```python
from build123d import *

# Parameters (mm, degrees)
F0_W     = 60
F0_H     = 9
F0_R     = 2
F1_DEPTH = 3
F3_DEPTH = 9
F5_DEPTH = 9


with BuildPart() as f1:
    # F0 (on Top) → F1 (new body)
    with BuildSketch(Plane.XY):
        Rectangle(F0_W, F0_H)
        with Locations((-14, 0)):
            Circle(F0_R, mode=Mode.SUBTRACT)
        with Locations((-7, 0)):
            Circle(F0_R, mode=Mode.SUBTRACT)
        Circle(F0_R, mode=Mode.SUBTRACT)
        with Locations((7, 0)):
            Circle(F0_R, mode=Mode.SUBTRACT)
        with Locations((14, 0)):
            Circle(F0_R, mode=Mode.SUBTRACT)
    extrude(amount=F1_DEPTH)

    # F2 (on face) → F3 (join)
    with BuildSketch(Plane(origin=(-30, 0, 0), x_dir=(0, -1, 0), z_dir=(-1, 0, 0))):
        with BuildLine():
            ThreePointArc((0, 0), (1.06066, 0.43934), (1.5, 1.5))
            ThreePointArc((1.5, 1.5), (1.06066, 2.56066), (0, 3))
            ThreePointArc((0, 3), (-1.5, 1.5), (0, 0))
        make_face()
    extrude(amount=F3_DEPTH)

    # F4 (on face) → F5 (join)
    with BuildSketch(Plane.YZ.offset(30)):
        with BuildLine():
            ThreePointArc((0, 0), (1.06066, 0.43934), (1.5, 1.5))
            ThreePointArc((1.5, 1.5), (1.06066, 2.56066), (0, 3))
            ThreePointArc((0, 3), (-1.5, 1.5), (0, 0))
        make_face()
    extrude(amount=F5_DEPTH)


solid = f1.part
```
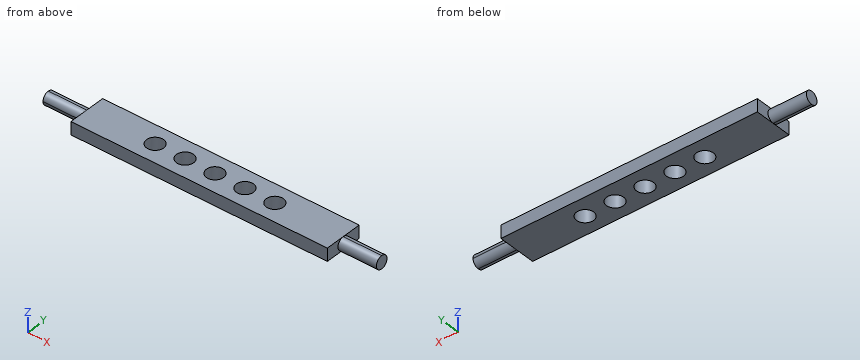
Part model, mm, in its own coordinate system. Round coordinates to 2 decimals unless told otherwise and drop trailing zeros. Loops run counter-clockwise (first coordinate to the right, second up) from the corner with the lowest first, then second, coordinate; pieces in that order, holes last.
1. Slice it at D-D (x = -33). Give the cut face in (y, z).
Solutions:
outline: circle Ø3 at (0, 1.5)
2. Flat gauge pin, fed straight in: pin 1 (5 mm diameter, centred on x = 14, y = 0, fed in from -Z). Where does the tip first touch, or does it go through?
Solutions:
pin 1: stops at z = 0
3. Slice it at A-A (x = -7). Give the cut face in (y, z).
Solutions:
outline: (-4.5, 0) - (-2, 0) - (-2, 3) - (-4.5, 3) - close; (2, 0) - (4.5, 0) - (4.5, 3) - (2, 3) - close
4. Slice it at C-C (y = -3.5). Give the cut face in (x, z).
Solutions:
outline: (-30, 0) - (30, 0) - (30, 3) - (-30, 3) - close
5. Drill centre lines: line 1 along X through (y, z) = (-0.25, 2.05); line 2 along Y through (x, z) = (14, 2.3); line 3 along X through (y, z) = (0.75, 2.5). Where is each one in solid material? Low to high.
Solutions:
line 1: x = -39 to -15.98, -12.02 to -8.98, -5.02 to -1.98, 1.98 to 5.02, 8.98 to 12.02, 15.98 to 39
line 2: y = -4.5 to -2, 2 to 4.5
line 3: x = -39 to -15.85, -12.15 to -8.85, -5.15 to -1.85, 1.85 to 5.15, 8.85 to 12.15, 15.85 to 39
6. Slice it at B-B (z = 0.6). Give the cut face in (x, y), and give its area (3 significant figures).
Solutions:
outline: (-39, -1.2) - (-30, -1.2) - (-30, -4.5) - (30, -4.5) - (30, -1.2) - (39, -1.2) - (39, 1.2) - (30, 1.2) - (30, 4.5) - (-30, 4.5) - (-30, 1.2) - (-39, 1.2) - close; hole circle Ø4 at (-14, 0); hole circle Ø4 at (-7, 0); hole circle Ø4 at (0, 0); hole circle Ø4 at (7, 0); hole circle Ø4 at (14, 0)
area: 520 mm2
